from build123d import *

# Parameters (mm, degrees)
F2_R     = 6.35
F3_DEPTH = 12.7


with BuildPart() as f1:
    # F0 (on Right) → F1 (revolve)
    with BuildSketch(Plane.YZ):
        Polygon((-254, 0), (0, 0), (0, 31.75), (-101.6, 31.75), (-101.6, 63.5), (-190.5, 63.5), (-190.5, 44.45), (-206.375, 44.45), (-238.125, 76.2), (-254, 76.2), align=None)
    revolve(axis=Axis((0, -127, 0), (0, 1, 0)))

    # F2 (on face) → F3 (join)
    with BuildSketch(Plane.XZ.offset(254)):
        with Locations((0, 63.5)):
            Circle(F2_R)
    extrude(amount=F3_DEPTH)


solid = f1.part
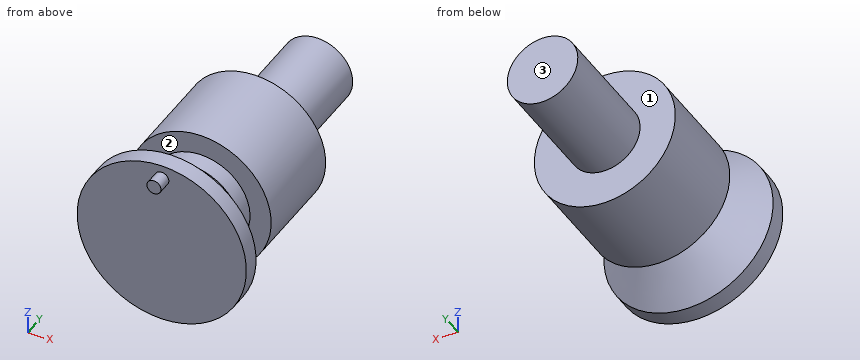
Here's how the part is built. I have some questions about the finished solid (model axes, mm). Face numbers are marked on the shaded views. A direction names the side the tool comes from. Coordinates: 2 decimals unless noted, no trailing zeros. Order: outer loops, then holes, each group sorted by start corner. A loop starts at its lowest first (then second) coordinate and runs counter-clockwise, first axis right, second up.
Item 1: If we section it at C-C on y = -34: List the corners of the cut face in (x, z) for me.
Result sheet:
outline: circle Ø63.5 at (0, 0)
Item 2: I need wall thicknesses on line 1 (Y direction, x = -53.5, z = 5); line 2 (Y direction, x = -43.5, z = 2); line 3 (Y direction, x = 0, z = 52.5) (3 decimals). Which ranges of each line are inside material? Lowest first, please.
Result sheet:
line 1: y = -254 to -215.66, -190.5 to -101.6
line 2: y = -254 to -101.6
line 3: y = -254 to -214.425, -190.5 to -101.6
Item 3: If we section it at A-A on x = 0: List the corners of the cut face in (y, z) for me (3 decimals).
Result sheet:
outline: (-266.7, 57.15) - (-254, 57.15) - (-254, -76.2) - (-238.125, -76.2) - (-206.375, -44.45) - (-190.5, -44.45) - (-190.5, -63.5) - (-101.6, -63.5) - (-101.6, -31.75) - (0, -31.75) - (0, 31.75) - (-101.6, 31.75) - (-101.6, 63.5) - (-190.5, 63.5) - (-190.5, 44.45) - (-206.375, 44.45) - (-238.125, 76.2) - (-254, 76.2) - (-254, 69.85) - (-266.7, 69.85) - close
Item 4: If we section it at B-B on z = 0: List the corners of the cut face in (x, y) for me (3 decimals).
Result sheet:
outline: (-76.2, -254) - (76.2, -254) - (76.2, -238.125) - (44.45, -206.375) - (44.45, -190.5) - (63.5, -190.5) - (63.5, -101.6) - (31.75, -101.6) - (31.75, 0) - (-31.75, 0) - (-31.75, -101.6) - (-63.5, -101.6) - (-63.5, -190.5) - (-44.45, -190.5) - (-44.45, -206.375) - (-76.2, -238.125) - close
Item 5: For the marked faces 1, 2 and 3, which set-ups out of +Z, -Z, +X, -X, +Y, -Y let a thin tool reach every point of the face, with its end or its side?
Result sheet:
face 1: +Y
face 2: none
face 3: +Z, -Z, +X, -X, +Y
Item 6: For P1, Ø12, axis at x = 35.5, z = 39.5, coming from the +Y side; P2, Ø2, axis at y = -71.5, z = 33, coming from the +X side; P3, Ø2, axis at x = -47.5, z = -25.5, coming from the -Y side; P4, Ø3, axis at y = -61.5, z = -30, coming from the -X side, each with a flat end and sliding along its axis, tell me the tip position at first contact or that it passes through.
Result sheet:
P1: stops at y = -101.6
P2: passes through
P3: stops at y = -254
P4: stops at x = -13.99
Item 7: If we section it at D-D on y = -161: List the corners of the cut face in (x, z) for me.
Result sheet:
outline: circle Ø127 at (0, 0)
